```python
from build123d import *

# Parameters (mm, degrees)
F1_DEPTH = 2.54


with BuildPart() as f1:
    # F0 (on Top) → F1 (new body)
    with BuildSketch(Plane.XY):
        with BuildLine():
            ThreePointArc((0, 48.26), (34.124973, 34.124973), (48.26, 0))
            Line((48.26, 0), (150.8125, 0))
            ThreePointArc((150.8125, 0), (106.183757, 106.183757), (0, 150.8125))
            Line((0, 150.8125), (0, 48.26))
        make_face()
        with BuildLine():
            Line((84.506493, 110.11853), (52.578475, 22.397019))
            ThreePointArc((52.578475, 22.397019), (49.801558, 28.034396), (46.422481, 33.332803))
            Line((46.422481, 33.332803), (76.52652, 116.04297))
            ThreePointArc((76.52652, 116.04297), (80.569209, 113.151738), (84.506493, 110.11853))
        make_face(mode=Mode.SUBTRACT)
        with BuildLine():
            Line((108.98855, 6.35), (98.852257, 6.35))
            Line((98.852257, 6.35), (120.71846, 66.4269))
            ThreePointArc((120.71846, 66.4269), (123.721116, 60.419279), (126.431564, 54.274287))
            Line((126.431564, 54.274287), (108.98855, 6.35))
        make_face(mode=Mode.SUBTRACT)
        with BuildLine():
            ThreePointArc((131.706002, 39.059832), (133.869559, 30.368774), (135.471763, 21.55694))
            Line((135.471763, 21.55694), (129.93689, 6.35))
            Line((129.93689, 6.35), (119.800596, 6.35))
            Line((119.800596, 6.35), (131.706002, 39.059832))
        make_face(mode=Mode.SUBTRACT)
        with BuildLine():
            Line((67.091871, 6.35), (56.796127, 6.35))
            Line((56.796127, 6.35), (91.779944, 103.885775))
            ThreePointArc((91.779944, 103.885775), (95.827883, 100.016544), (99.717507, 95.988197))
            Line((99.717507, 95.988197), (67.091871, 6.35))
        make_face(mode=Mode.SUBTRACT)
        with BuildLine():
            Line((88.040211, 6.35), (77.903917, 6.35))
            Line((77.903917, 6.35), (107.29494, 87.10117))
            ThreePointArc((107.29494, 87.10117), (110.755392, 82.487904), (114.022499, 77.735749))
            Line((114.022499, 77.735749), (88.040211, 6.35))
        make_face(mode=Mode.SUBTRACT)
        with BuildLine():
            ThreePointArc((21.763532, 52.843838), (17.280179, 54.474929), (12.676404, 55.726397))
            Line((12.676404, 55.726397), (41.041329, 133.658389))
            ThreePointArc((41.041329, 133.658389), (45.538899, 132.089902), (49.980383, 130.368999))
            Line((49.980383, 130.368999), (21.763532, 52.843838))
        make_face(mode=Mode.SUBTRACT)
        with BuildLine():
            Line((31.26083, 136.49254), (6.35, 68.050598))
            Line((6.35, 68.050598), (6.35, 95.899834))
            Line((6.35, 95.899834), (21.858168, 138.508175))
            ThreePointArc((21.858168, 138.508175), (26.576847, 137.581285), (31.26083, 136.49254))
        make_face(mode=Mode.SUBTRACT)
        with BuildLine():
            ThreePointArc((38.763073, 41.994603), (34.94125, 45.224236), (30.851582, 48.107197))
            Line((30.851582, 48.107197), (59.269677, 126.185272))
            ThreePointArc((59.269677, 126.185272), (63.546378, 123.975746), (67.744416, 121.620189))
            Line((67.744416, 121.620189), (38.763073, 41.994603))
        make_face(mode=Mode.SUBTRACT)
    extrude(amount=F1_DEPTH)

    # F2: F1 across plane


with BuildPart() as f1_1:
    add(f1.part)
    add(f1.part.mirror(Plane.YZ))


solid = f1_1.part
```
Verification items for the finished model (mm, model axes). A direction names the side the tool comes from. Coordinates: 2 decimals unless noted, no trailing zeros. Order: outer loops, then holes, each group sorted by start corner. A loop starts at its lowest first (then second) coordinate and runs counter-clockwise, first axis right, second up. Notation, with made-up numbers: (8.5, 70.25) -> (56.5, 70.25) arc R23 cw to (56.5, 96.25) -> close; hole circle Ø8 at (42, 22.25). An arc over 180 degrees is marked (long way). Put each result on its own line as item: value. Start each with the question number.
1) Tool access check on faces 1 (the cylindrical face through (107.347, 105.008, 1.252)), 2 (the flat face through (-44.86, 86.6, 1.25)). Record the directions out of +Z, -Z, +X, -X, +Y, -Y that give a thin tool (end or side, any length) a straight path to the whole face; none if there is none.
2) Go/stop test with flat-tipped pins: pin 1 (12 mm diameter, centred on x = -7.5, y = 48.5, fed in from -Z); pin 2 (0.8 mm diameter, centred on y = 83, z = 1, fed in from -X); pin 3 (1.3 mm diameter, centred on x = 84.5, z = 1, fed in from +Y); pin 4 (0.8 mm diameter, centred on x = -80.5, z = 1, fed in from +Y). Record where each tip stops, or that it passes through.
3) Material ranges on L1, parallel to X at y = 127, z = 1.8; L2, parallel to Y at x = -138, z = 1; L3, parallel to Y at x = 138.5, z = 0.1, recorded low to high.
4) Cross-section at A-A (x = -34.5). Enter the section's corners in (y, z), plus the area to 3 significant figures.
5) Cross-section at B-B (z = 1). State how many separate pieces and enclosed holes the cut face has, plus the area to 3 significant figures.
Geometry check:
1. face 1: +Z, -Z, +X, +Y
1. face 2: +Z, -Z
2. pin 1: stops at z = 0
2. pin 2: stops at x = -125.46
2. pin 3: stops at y = 124.63
2. pin 4: stops at y = 127.08
3. L1: x = -80.23 to -48.75, -38.62 to -27.81, -17.67 to 17.67, 27.81 to 38.62, 48.75 to 80.23
3. L2: y = 0 to 59.6
3. L3: y = 0 to 58.45
4. outline: (33.75, 0) -> (45.56, 0) -> (45.56, 2.54) -> (33.75, 2.54) -> close; (58.13, 0) -> (87.84, 0) -> (87.84, 2.54) -> (58.13, 2.54) -> close; (115.69, 0) -> (146.49, 0) -> (146.49, 2.54) -> (115.69, 2.54) -> close
4. area: 184 mm^2
5. separate pieces: 1
5. enclosed holes: 16
5. area: 20,700 mm^2
